Input: part model. Units: mm. Frame: model coordinates. A direction names the side the tool comes from. Coordinates: 2 decimals unless noted, no trailing zeros. Order: outer loops, then holes, each group sorted by start corner. A loop starts at its lowest first (then second) coordinate and runs counter-clockwise, first axis right, second up.
from build123d import *

# Parameters (mm, degrees)
SKETCH_1_W           = 10
SKETCH_1_H           = 30
EXTRUDE_1_DEPTH      = 5
SKETCH_2_W           = 15
SKETCH_2_H           = 30
EXTRUDE_2_DEPTH      = 5
SKETCH_4_R           = 1.5
CUT_EXTRUDE_1_DEPTH  = 21.615528128
EXTRUDE_3_DEPTH      = 5
EXTRUDE_3_DEPTH_BACK = 5
SKETCH_3_R           = 1.5
CUT_EXTRUDE_2_DEPTH  = 5
FILLET_1_R           = 1
FILLET_2_R           = 1


with BuildPart() as part:
    # 草圖1 → 填料-伸長1 (new body)
    with BuildSketch(Plane.XY):
        Rectangle(SKETCH_1_W, SKETCH_1_H)
    extrude(amount=EXTRUDE_1_DEPTH)

    # 草圖2 → 填料-伸長2 (add)
    with BuildSketch(Plane(origin=(5, 0, 0), x_dir=(0, 0, -1), z_dir=(1, 0, 0))):
        with Locations((-7.5, 0)):
            Rectangle(SKETCH_2_W, SKETCH_2_H)
    extrude(amount=EXTRUDE_2_DEPTH)

    # 草圖4 → 除料-伸長1 (cut, through all)
    with BuildSketch(Plane.XY.offset(5)):
        with Locations((0, 11)):
            Circle(SKETCH_4_R)
        with Locations((0, -11)):
            Circle(SKETCH_4_R)
    extrude(amount=-CUT_EXTRUDE_1_DEPTH, mode=Mode.SUBTRACT)

    # 草圖5 → 填料-伸長3 (add, two sides: drawn at the far end of the back side and taken through both)
    with BuildSketch(Plane.XZ.offset(-EXTRUDE_3_DEPTH_BACK)):
        Polygon((5, 15), (-5, 5), (5, 5), align=None)
    extrude(amount=EXTRUDE_3_DEPTH + EXTRUDE_3_DEPTH_BACK)

    # 草圖3 → 除料-伸長2 (cut)
    with BuildSketch(Plane.ZY.offset(-5)):
        with Locations(Location((10, 11, 0), (0, 0, 270))):
            Circle(SKETCH_3_R)
        with Locations(Location((10, -11, 0), (0, 0, 270))):
            Circle(SKETCH_3_R)
    extrude(amount=-CUT_EXTRUDE_2_DEPTH, mode=Mode.SUBTRACT)

    # 圓角1
    fillet_1_edges = [part.edges().sort_by_distance(p)[0] for p in [
        (10, 0, 0),
        (-1.5, 11, 0),
        (-1.5, -11, 0),
        (2.5, -15, 0),
        (-5, 0, 0),
        (2.5, 15, 0),
    ]]
    fillet(fillet_1_edges, radius=FILLET_1_R)

    # 圓角2
    # the kernel refuses this fillet: 1 mm, written as the material it adds along each edge
    with BuildSketch(Plane(origin=(-5, -5, 5), x_dir=(0, -1, 0), z_dir=(1, 0, 0))) as fillet_2_piece_1_section:
        with BuildLine():
            CenterArc((FILLET_2_R, -FILLET_2_R), FILLET_2_R, 90, 90)
            Line((0, -FILLET_2_R), (0, 0))
            Line((0, 0), (FILLET_2_R, 0))
        make_face()
    fillet_2_piece_1 = extrude(amount=12.5, mode=Mode.PRIVATE)
    fillet_2_piece_1 = split(fillet_2_piece_1, bisect_by=Plane(origin=(-2.333551082, -5.229183037, 7.666448918), z_dir=(0.7071067811865476, 0, -0.7071067811865475)), keep=Keep.TOP, mode=Mode.PRIVATE)
    add(fillet_2_piece_1)
    with BuildSketch(Plane(origin=(5, -5, 2.5), x_dir=(0, -1, 0), z_dir=(0, 0, 1))) as fillet_2_piece_2_section:
        with BuildLine():
            CenterArc((FILLET_2_R, -FILLET_2_R), FILLET_2_R, 90, 90)
            Line((0, -FILLET_2_R), (0, 0))
            Line((0, 0), (FILLET_2_R, 0))
        make_face()
    fillet_2_piece_2 = extrude(amount=12.5, mode=Mode.PRIVATE)
    fillet_2_piece_2 = split(fillet_2_piece_2, bisect_by=Plane(origin=(-0.738197557, -5.226395114, 9.261802443), z_dir=(0.7071067811865476, 0, -0.7071067811865475)), keep=Keep.TOP, mode=Mode.PRIVATE)
    add(fillet_2_piece_2)
    with BuildSketch(Plane(origin=(-5, 5, 5), x_dir=(0, 1, 0), z_dir=(1, 0, 0))) as fillet_2_piece_3_section:
        with BuildLine():
            CenterArc((FILLET_2_R, FILLET_2_R), FILLET_2_R, 180, 90)
            Line((0, FILLET_2_R), (0, 0))
            Line((0, 0), (FILLET_2_R, 0))
        make_face()
    fillet_2_piece_3 = extrude(amount=12.5, mode=Mode.PRIVATE)
    fillet_2_piece_3 = split(fillet_2_piece_3, bisect_by=Plane(origin=(-2.333551082, 5.229183037, 7.666448918), z_dir=(0.7071067811865476, 0, -0.7071067811865475)), keep=Keep.TOP, mode=Mode.PRIVATE)
    add(fillet_2_piece_3)
    with BuildSketch(Plane(origin=(5, 5, 2.5), x_dir=(0, 1, 0), z_dir=(0, 0, 1))) as fillet_2_piece_4_section:
        with BuildLine():
            CenterArc((FILLET_2_R, FILLET_2_R), FILLET_2_R, 180, 90)
            Line((0, FILLET_2_R), (0, 0))
            Line((0, 0), (FILLET_2_R, 0))
        make_face()
    fillet_2_piece_4 = extrude(amount=12.5, mode=Mode.PRIVATE)
    fillet_2_piece_4 = split(fillet_2_piece_4, bisect_by=Plane(origin=(-0.738197557, 5.226395114, 9.261802443), z_dir=(0.7071067811865476, 0, -0.7071067811865475)), keep=Keep.TOP, mode=Mode.PRIVATE)
    add(fillet_2_piece_4)


solid = part.part
Item 1: Pin query (flat end, axial travel): pin 1 Ø1 at (y, z) = (7.5, 13) entering from -X; pin 2 Ø5 at (x, y) = (0, 11) entering from +Z; pin 3 Ø4 at (x, z) = (0.5, 9) entering from -Y; pin 4 Ø4 at (y, z) = (11, 10) entering from +X. Return the tip coordinate at first contact, or that it passes through.
Response values:
pin 1: stops at x = 5
pin 2: stops at z = 5
pin 3: stops at y = -5
pin 4: stops at x = 10
Item 2: Cut plane D-D on y = -2.5. Return loops of the section in (x, z).
Response values:
outline: (-5, 1) arc R1 ccw to (-4, 0) - (9, 0) arc R1 ccw to (10, 1) - (10, 15) - (5, 15) - (-5, 5) - close
Item 3: Access query for faces 5 (the face through (-0.325, 9.536, 3.028)), 6 (the face through (4.699, 5.285, 9.93)), 7 (the face through (-0.07, -5.301, 5.285)). Directions: +Z, -Z, +X, -X, +Y, -Y. A direction counts if a zero-diameter tool reaches every point of the face in a straight line with its end or side. Return the directions, or none.
Response values:
face 5: +Z, -Z
face 6: +Z, -X, +Y
face 7: +Z, -X, -Y
Item 4: Cut plane A-A on y = 11. Return loops of the section in (x, z), then the cut area to 3 significant figures.
Response values:
outline: (-5, 1) arc R1 ccw to (-4, 0) - (-2.5, 0) arc R1 ccw to (-1.5, 1) - (-1.5, 5) - (-5, 5) - close; (1.5, 1) arc R1 ccw to (2.5, 0) - (9, 0) arc R1 ccw to (10, 1) - (10, 8.5) - (5, 8.5) - (5, 5) - (1.5, 5) - close; (5, 11.5) - (10, 11.5) - (10, 15) - (5, 15) - close
area: 94.1 mm2
Item 5: Cut plane B-B on x = 0. Return loops of the section in (y, z).
Response values:
outline: (-15, 1) arc R1 ccw to (-14, 0) - (-13.5, 0) arc R1 ccw to (-12.5, 1) - (-12.5, 5) - (-15, 5) - close; (-9.5, 1) arc R1 ccw to (-8.5, 0) - (8.5, 0) arc R1 ccw to (9.5, 1) - (9.5, 5) - (6, 5) arc R1 cw to (5, 6) - (5, 10) - (-5, 10) - (-5, 6) arc R1 cw to (-6, 5) - (-9.5, 5) - close; (12.5, 1) arc R1 ccw to (13.5, 0) - (14, 0) arc R1 ccw to (15, 1) - (15, 5) - (12.5, 5) - close
Item 6: Ray query, probe 1 along Y at (x, z) = (-0.75, 3); probe 2 along Z at (x, y) = (7.25, 11); probe 3 along Y at (x, z) = (1, 2.5). Return the intervals inside material, ascending.
Response values:
probe 1: y = -15 to -12.3, -9.7 to 9.7, 12.3 to 15
probe 2: z = 0 to 8.5, 11.5 to 15
probe 3: y = -15 to -12.12, -9.88 to 9.88, 12.12 to 15
Item 7: Draft query along X for faces 1 (the face through (9.715, 0.21, 0.301)), 2 (the face through (-0.325, -12.464, 3.028)), 3 (the face through (5, 9.6, 11.2)), 4 (the face through (2.605, -14.715, 0.301)). Return one class per face: pulls with the +X half, pulls with the -X half, needs draft (parallel to the pull), parting line crosses it, or undercut.
Response values:
face 1: pulls with the +X half
face 2: undercut
face 3: pulls with the -X half
face 4: needs draft
Item 8: Cut plane C-C on z = 10. Return loops of the section in (x, y).
Response values:
outline: (0, -5) - (4, -5) arc R1 cw to (5, -6) - (5, -9.5) - (10, -9.5) - (10, 9.5) - (5, 9.5) - (5, 6) arc R1 cw to (4, 5) - (0, 5) - close; (5, -15) - (10, -15) - (10, -12.5) - (5, -12.5) - close; (5, 12.5) - (10, 12.5) - (10, 15) - (5, 15) - close
